```python
from build123d import *

# Parameters (mm, degrees)
SKETCH2_R          = 1.25
CUT_EXTRUDE1_DEPTH = 10


with BuildPart() as part:
    # Sketch1 → Revolve1 (revolve)
    with BuildSketch(Plane.XY, mode=Mode.PRIVATE) as revolve1_sk:
        Polygon((0, 0), (0, -1.5), (2, -1.5), (2, -9.5), (3, -9.5), (6.85, -1.5), (14.1, -1.5), (14.1, 0), align=None)
    revolve(revolve1_sk.sketch.rotate(Axis((0, 0, 0), (0, -1, 0)), 90), axis=Axis((0, 0, 0), (0, -1, 0)))

    # Sketch2 → Cut-Extrude1 (cut)
    with BuildSketch(Plane.XY):
        with Locations((0, -5.6)):
            Circle(SKETCH2_R)
    extrude(amount=-CUT_EXTRUDE1_DEPTH, mode=Mode.SUBTRACT)


solid = part.part
```
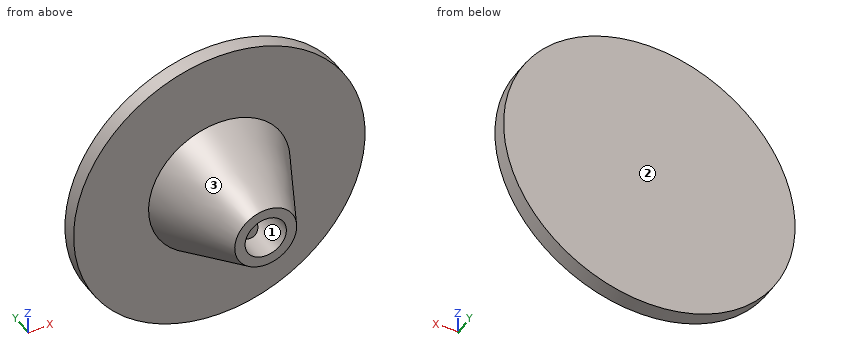
Can you work these out from the model? Positions are in its coordinate system, mm. Face numbers are marked on the shaded views. Coordinates: 2 decimals unless noted, no trailing zeros. Loops run counter-clockwise (first coordinate to the right, second up) from the corner with the lowest first, then second, coordinate; pieces in that order, holes last.
Item 1: Please list where these lines run through material, in increasing order: L1, parallel to Y at x = -7.25, z = 1.5; L2, parallel to X at y = -7, z = -0.5; L3, parallel to X at y = -2.75, z = -1.25.
Answers below:
L1: y = -1.5 to 0
L2: x = -4.17 to -1.94, 1.94 to 4.17
L3: x = -6.12 to -1.56, 1.56 to 6.12
Item 2: I'm going to push flat-ended pins straight in: pin 1 (1 mm diameter, centred on x = -3, y = -6.5, fed in from -Z); pin 2 (2 mm diameter, centred on y = -1, z = 2.5, fed in from +X); pin 3 (14 mm diameter, centred on x = 4.5, z = -6, fed in from -Y); pin 4 (2 mm diameter, centred on x = 5.5, y = -3, fed in from +Z). Where does each tip first touch, or does it pass through?
Answers below:
pin 1: stops at z = -3.78
pin 2: stops at x = 14.02
pin 3: stops at y = -9.5
pin 4: stops at z = 4.37
Item 3: If we mould it in two halves opening along X, with no side actions, what happens to the marked faces 1, 2 and 3? For each: released by +X, released by -X, zero draft, split by the parting line, or undercut.
Answers below:
face 1: undercut
face 2: zero draft
face 3: split by the parting line
Item 4: Suppose I cut it at B-B (z = 0). Please give me the cut outline in (x, y).
Answers below:
outline: (-14.1, -1.5) - (-6.85, -1.5) - (-3, -9.5) - (-2, -9.5) - (-2, -1.5) - (2, -1.5) - (2, -9.5) - (3, -9.5) - (6.85, -1.5) - (14.1, -1.5) - (14.1, 0) - (-14.1, 0) - close
Item 5: Suppose I cut it at D-D (y = -8). Please give me the cut outline in (x, z), then the cut area to 3 significant figures.
Answers below:
outline: circle Ø7.44 at (0, 0); hole circle Ø4 at (0, 0)
area: 31.0 mm2
Item 6: Suppose I cut it at A-A (x = 0). Please give me the cut outline in (y, z), then the cut area to 3 significant figures.
Answers below:
outline: (-9.5, -3) - (-6.85, -4.28) - (-6.85, -2) - (-9.5, -2) - close; (-9.5, 2) - (-1.5, 2) - (-1.5, -2) - (-4.35, -2) - (-4.35, -5.48) - (-1.5, -6.85) - (-1.5, -14.1) - (0, -14.1) - (0, 14.1) - (-1.5, 14.1) - (-1.5, 6.85) - (-9.5, 3) - close
area: 81.9 mm2
Item 7: Suppose I cut it at C-C (y = -1). Please give me the cut outline in (x, z).
Answers below:
outline: circle Ø28.2 at (0, 0)
